Could you check a few things on this drawing? It's one solid part, dimensions in mm from its lowest x, y, z. A direction names the side the tool comes from. Round coordinates to 2 decimals unless told otherwise and drop trailing zeros. Loops run counter-clockwise (first coordinate to the right, second up) from the corner with the lowest first, then second, coordinate; pieces in that order, holes last. Notation, with made-up numbers: M -7,-13.75 L 49,-13.75 A14 cw 49,-1.75 Z; hole C 39,-21 d1. An arc over 180 degrees is marked long. Answer as a JSON object with one key per item and string values.
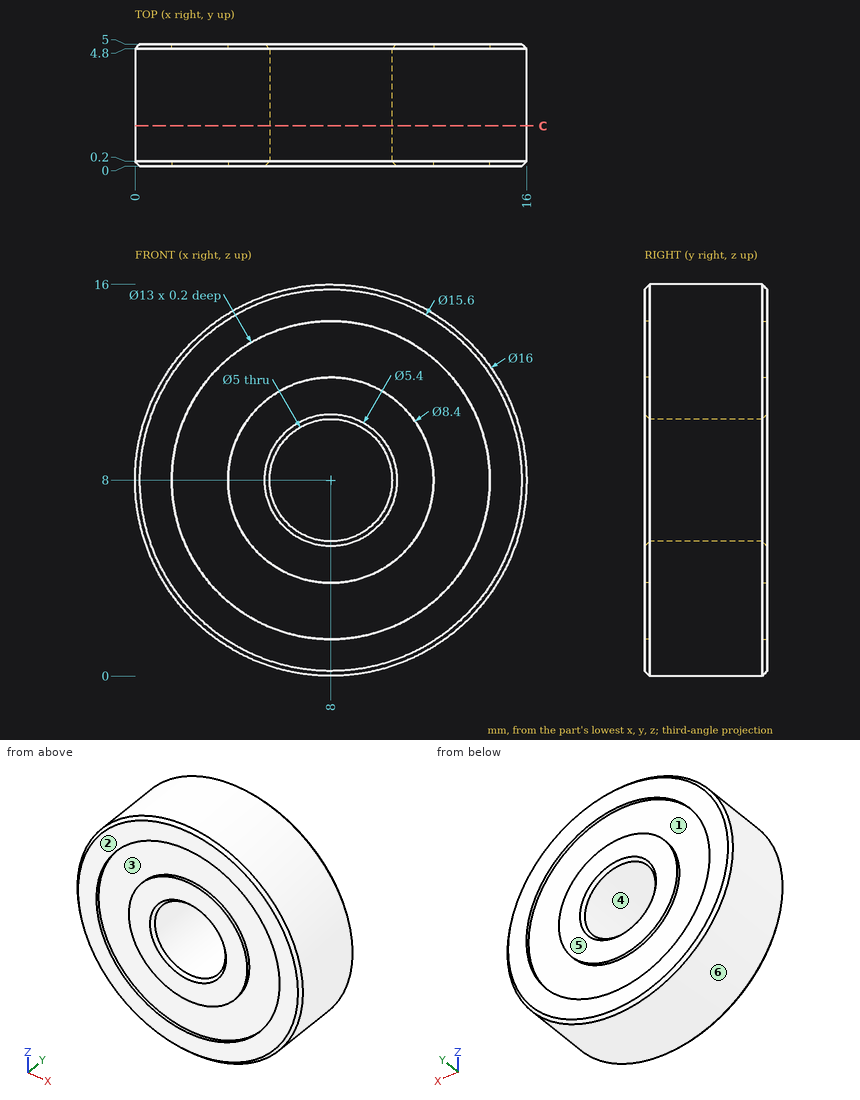
Item 1: If we mould it in two halves opening along X, with no side actions, what happens to the marked faces 4, 5 and 6? For each: pulls with the +X half, pulls with the -X half, needs draft (parallel to the pull), parting line crosses it, or undercut.
Resolved:
{"face 4": "undercut", "face 5": "needs draft", "face 6": "parting line crosses it"}
Item 2: I want a section at C-C, the plane y = 1.65. Please give me the cut outline in (x, z), then the cut area to 3 significant figures.
Resolved:
{"outline": "C 8,8 d16; hole C 8,8 d5", "area": "181 mm²"}
Item 3: I'm going to push flat-ended pins straight in: pin 1 Ø3 at (x, y) = (7.5, 2.5) entering from -Z; pin 2 Ø1.5 at (y, z) = (4.5, 4) entering from +X; pin 3 Ø1.5 at (y, z) = (4.5, 4) entering from -X; pin 4 Ø1 at (x, y) = (9.5, 1) entering from +Z. Where does each tip first touch, or does it pass through?
Resolved:
{"pin 1": "z = 0", "pin 2": "x = 15.31", "pin 3": "x = 0.69", "pin 4": "z = 15.94"}
Item 4: Please list where these lines run through material, in increasing order: probe 1 along Z at (x, y) = (8, 0.1); probe 2 along Z at (x, y) = (8, 4.95); probe 3 along X at (y, z) = (3.05, 8). Write a range as from..to.
Resolved:
{"probe 1": "0.1..1.5, 3.8..5.4, 10.6..12.2, 14.5..15.9", "probe 2": "0.15..1.5, 3.8..5.35, 10.65..12.2, 14.5..15.85", "probe 3": "0..5.5, 10.5..16"}
Item 5: On a 3-axis mill with a long thin cutter (end or side, diameter ignored), from which of +Z, -Z, +X, -X, +Y, -Y can I reach the whole of each face in a straight line? I mean the marked faces 1, 2 and 3. Say none if no direction works.
Resolved:
{"face 1": "+Y", "face 2": "+Z, -Z, +X, -X, -Y", "face 3": "-Y"}
